```python
from build123d import *

# Parameters (mm, degrees)
SKETCH3_R          = 6.9
CUT_EXTRUDE1_DEPTH = 6
SKETCH4_R          = 6.9
CUT_EXTRUDE2_DEPTH = 6
CUT_EXTRUDE3_DEPTH = 8.15


with BuildPart() as part:
    # Sketch1 → Revolve1 (revolve)
    with BuildSketch(Plane.XY, mode=Mode.PRIVATE) as revolve1_sk:
        Polygon((2.25, 9), (4, 9), (4, 0.5), (4.5, 0), (7.65, 0), (8.15, 0.5), (8.15, 7.5), (7.6, 7.5), (7.6, 9.15), (6.85, 9.15), (6.85, 12.2), (7.6, 12.2), (7.6, 14.5), (4, 14.5), (4, 10.5), (2.25, 10.5), align=None)
    revolve(revolve1_sk.sketch.rotate(Axis((0, 0, 0), (0, 1, 0)), 270), axis=Axis((0, 0, 0), (0, 1, 0)))

    # Sketch2 → Revolve2 (revolve)
    with BuildSketch(Plane(origin=(0, 0, 0), x_dir=(0, 0, -1), z_dir=(1, 0, 0)), mode=Mode.PRIVATE) as revolve2_sk:
        Polygon((4.75, 14.5), (7.5, 14.5), (7.5, 17.9), (7.15, 17.9), (7.15, 19), (7.5, 19), (7.5, 19.4), (7, 19.9), (5.25, 19.9), (4.75, 19.4), align=None)
    revolve(revolve2_sk.sketch.rotate(Axis((0, 14.5, 0), (0, 1, 0)), 180), axis=Axis((0, 14.5, 0), (0, 1, 0)))

    # Sketch3 → Cut-Extrude1 (cut)
    with BuildSketch(Plane(origin=(0, 14.5, 0), x_dir=(1, 0, 0), z_dir=(0, 1, 0))):
        with Locations((7.25, 0)):
            Circle(SKETCH3_R)
    extrude(amount=CUT_EXTRUDE1_DEPTH, mode=Mode.SUBTRACT)

    # Sketch4 → Cut-Extrude2 (cut)
    with BuildSketch(Plane(origin=(0, 14.5, 0), x_dir=(1, 0, 0), z_dir=(0, 1, 0))):
        with Locations((-7.25, 0)):
            Circle(SKETCH4_R)
    extrude(amount=CUT_EXTRUDE2_DEPTH, mode=Mode.SUBTRACT)

    # Sketch5 → Cut-Revolve1 (revolve, cut)
    with BuildSketch(Plane(origin=(0, 3.6, 0), x_dir=(1, 0, 0), z_dir=(0, 1, 0)), mode=Mode.PRIVATE) as cut_revolve1_sk:
        Polygon((6, 6.55), (7.0065, 6.55), (7.0065, 0.3), (7.25, 0.3), (7.25, -2.6), (8.5, -2.6), (8.5, -8.15), (6, -8.15), align=None)
    revolve(cut_revolve1_sk.sketch.rotate(Axis((6, 3.6, 8.15), (0, 0, -1)), 180), axis=Axis((6, 3.6, 8.15), (0, 0, -1)), mode=Mode.SUBTRACT)

    # Sketch6 → Cut-Extrude3 (cut)
    with BuildSketch(Plane(origin=(0, 0, 0), x_dir=(0, 0, -1), z_dir=(1, 0, 0))):
        with BuildLine():
            Line((-0.3, 19.9), (-0.3, 0))
            Line((-0.3, 0), (0.3, 0))
            Line((0.3, 0), (0.3, 19.9))
            ThreePointArc((0.3, 19.9), (0, 20.2), (-0.3, 19.9))
        make_face()
    extrude(amount=CUT_EXTRUDE3_DEPTH, mode=Mode.SUBTRACT)


solid = part.part
```
The model under review builds one solid part; all positions refer to its coordinate system, in mm. A direction names the side the tool comes from. Round coordinates to 2 decimals unless told otherwise and drop trailing zeros. Loops run counter-clockwise (first coordinate to the right, second up) from the corner with the lowest first, then second, coordinate; pieces in that order, holes last. Notation, with made-up numbers: (19, 76.5) -> (76, 76.5) arc R12 ccw to (76, 81.5) -> close; hole circle Ø1 at (38, 10.5). An arc over 180 degrees is marked (long way). Answer as a JSON object with one key per item and string values. Group by question number.
1) We need section C-C on y = 3.6. Write out the cut boundary in (x, z).
2) For pin 1 Ø8 at (x, y) = (-1.5, 14.5) entering from -Z; pin 2 Ø8 at (x, y) = (6, 3.6) entering from +Z; pin 3 Ø4 at (x, z) = (-0.5, -0.5) entering from +Y; pin 4 Ø3.5 at (x, z) = (0, 0) entering from -Y, all flat-tipped, find the tip position at first contact; note any pin that passes through.
3) We need section D-D on y = 16.25. Write out the cut boundary in (x, z), then the cut area to 3 significant figures.
4) For faces 1 (the face through (-2, 10.5, 2)), 2 (the face through (-0.06, 18.46, 7.15)), 3 (the face through (-2.98, 17.16, 5.42)), 4 (the face through (6, 7, -0.3)), 5 (the face through (6, 9.15, -4)), list the 3-axis set-ups (+Z, -Z, +X, -X, +Y, -Y) from which the entire face can be reached by the end or side of a thin tool; tool diameter is ignored.
5) We need section A-A on y = 18.75. Write out the cut boundary in (x, z).
6) We need section B-B on z = 0. Write out the cut boundary in (x, y).
7) For line 1 (Z direction, x = 0, y = 11.8); line 2 (Z direction, x = 0, y = 10.25); line 3 (X direction, y = 3.75, z = 2), list the stretches that pass through material, from the lowest coordinate up. Write a range as [from, to].
8) Mouldability with a two-part tool opening along Z and no side actions: class faces 6 (the face through (0.02, 17.9, 7.3)), 7 (the face through (0.06, 18.46, -7.15)), 8 (the face through (-0.03, 16.92, 4.75)) as released by +Z, released by -Z, zero draft, split by the parting line, or undercut.
Result set:
{
 "1": {"outline": "(3.5, 2.6) -> (3.5, 7.36) arc R8.15 ccw (long way) to (4.99, -6.44) -> (4.99, -0.3) -> (3.99, -0.3) arc R4 cw (long way) to (3.99, 0.3) -> (4.75, 0.3) -> (4.75, 2.6) -> close; (7.01, -4.16) arc R8.15 ccw to (8.14, -0.3) -> (7.01, -0.3) -> close; (7.25, 0.3) -> (8.14, 0.3) arc R8.15 ccw to (7.72, 2.6) -> (7.25, 2.6) -> close"},
 "2": {"pin 1": "z = -7.6", "pin 2": "z = 7.9", "pin 3": "y = 10.5", "pin 4": "through"},
 "3": {"outline": "(-4.22, -6.2) arc R7.5 ccw to (4.22, -6.2) arc R6.9 cw to (1.9, -4.35) arc R4.75 cw to (-1.9, -4.35) arc R6.9 cw to start; (-4.22, 6.2) arc R6.9 cw to (-1.9, 4.35) arc R4.75 cw to (1.9, 4.35) arc R6.9 cw to (4.22, 6.2) arc R7.5 ccw to start", "area": "34.2 mm²"},
 "4": {"face 1": "+Y", "face 2": "+Z", "face 3": "-X, +Y", "face 4": "+X, +Y, -Y", "face 5": "none"},
 "5": {"outline": "(-3.87, -6.01) arc R7.15 ccw to (3.87, -6.01) arc R6.9 cw to (1.9, -4.35) arc R4.75 cw to (-1.9, -4.35) arc R6.9 cw to start; (-3.87, 6.01) arc R6.9 cw to (-1.9, 4.35) arc R4.75 cw to (1.9, 4.35) arc R6.9 cw to (3.87, 6.01) arc R7.15 ccw to start"},
 "6": {"outline": "(-8.15, 0.5) -> (-7.65, 0) -> (-4.5, 0) -> (-4, 0.5) -> (-4, 9) -> (-2.25, 9) -> (-2.25, 10.5) -> (-4, 10.5) -> (-4, 14.5) -> (-7.6, 14.5) -> (-7.6, 12.2) -> (-6.85, 12.2) -> (-6.85, 9.15) -> (-7.6, 9.15) -> (-7.6, 7.5) -> (-8.15, 7.5) -> close"},
 "7": {"line 1": "[-6.85, -4], [4, 6.85]", "line 2": "[-6.85, -2.25], [2.25, 6.85]", "line 3": "[-7.9, -3.46], [3.46, 4.76], [7.24, 7.9]"},
 "8": {"face 6": "zero draft", "face 7": "released by -Z", "face 8": "undercut"}
}
